Part model, mm, in its own coordinate system. Face numbers are marked on the shaded views. A direction names the side the tool comes from. Coordinates: 2 decimals unless noted, no trailing zeros. Order: outer loops, then holes, each group sorted by start corner. A loop starts at its lowest first (then second) coordinate and runs counter-clockwise, first axis right, second up.
1) Cut at B-B (x = -20.5). List the corners of the cut face in (y, z) (3 decimals), and give its area (3 significant figures).
2) Cut at D-D (x = -5.5). List the corners of the cut face in (y, z) (3 decimals).
3) Cut at C-C (y = 30.5). List the corners of the cut face in (x, z) (3 decimals), and give its area (3 significant figures).
4) Wall check: L1, parallel to Y at x = 12.5, z = 3; L2, parallel to Z at x = -19, y = 7; L3, parallel to X at y = 42.5, z = 4.5. Give the ranges that are in metal, low to high.
5) Mould opens along X. For the marked faces 1, 2 and 3 say: +X half, -X half, draft (parallel to the pull), parting line (faces both ways), or undercut.
6) Cut at A-A (y = -37.5). List the corners of the cut face in (x, z) (3 decimals), and give its area (3 significant figures).
7) Tool access for the marked faces 4, 5 and 6: list every direction of +Z, -Z, +X, -X, +Y, -Y with a clear straight run to the whole face (end or side of a thin tool).
8) Pin check, flat tips, straight feed: pin 1 Ø3 at (x, y) = (17.5, -5) entering from +Z (3 decimals); pin 2 Ø8 at (x, z) = (-1.5, 19) entering from -Y; pin 3 Ø1 at (y, z) = (-7.5, 24) entering from -X; pin 4 Ø12 at (x, y) = (-15.17, -34.82) entering from -Z. Stop position of each tip, or through.
```python
from build123d import *

# Parameters (mm, degrees)
F0_W      = 63.5
F0_H      = 101.6
F1_DEPTH  = 12.7
F5_DEPTH  = 6.35
F6_R      = 5.08
F8_D      = 10.16
F8_DEPTH  = 6.35
F8_TIP    = 3.0523719447
F10_D     = 15.24
F10_DEPTH = 12.7
F10_TIP   = 4.578557917
F12_DEPTH = 25.4
F13_R     = 5.08
F14_SIZE  = 1.905
F15_SIZE  = 1.905


with BuildPart() as f1:
    # F0 (on Top) → F1 (new body)
    with BuildSketch(Plane.XY):
        Rectangle(F0_W, F0_H)
    extrude(amount=F1_DEPTH)

    # F4 (on face) → F5 (join)
    with BuildSketch(Plane(origin=(-7.7671213914, -9.6767273995, 10.4118445509), x_dir=(0.8775350605, -0.3264402976, 0.3512391632), z_dir=(-0.4795124792, -0.5974042778, 0.6427876097))):
        Polygon((11.0284127295, 38.4279564023), (-4.4907014817, 5.8724405244), (24.646670238, -9.5275499275), (40.752428482, 24.2586095854), align=None)
    extrude(amount=-F5_DEPTH)

    # F6
    f6_edges = [f1.edges().sort_by_distance(p)[0] for p in [
        (3.43315, 16.768092, 38.405412),
        (29.517016, -3.313961, 39.199507),
    ]]
    fillet(f6_edges, radius=F6_R)

    # F8
    with Locations(Plane(origin=(-7.7671213914, -9.6767273995, 10.4118445509), x_dir=(0.8775350605, -0.3264402976, 0.3512391632), z_dir=(-0.4795124792, -0.5974042778, 0.6427876097))):
        with Locations((21.2519261986, 21.5889699757)):
            Hole(F8_D / 2, depth=F8_DEPTH)
            with Locations((0, 0, -(F8_DEPTH + F8_TIP / 2))):  # 118° drill point
                Cone(0, F8_D / 2, F8_TIP, mode=Mode.SUBTRACT)

    # F10
    with Locations(Plane.XY.offset(12.7)):
        with Locations((-15.1724275202, -34.8201803863)):
            Hole(F10_D / 2, depth=F10_DEPTH)
            with Locations((0, 0, -(F10_DEPTH + F10_TIP / 2))):  # 118° drill point
                Cone(0, F10_D / 2, F10_TIP, mode=Mode.SUBTRACT)

    # F11 (on face) → F12 (cut)
    with BuildSketch(Plane.XY.offset(12.7)):
        with BuildLine():
            ThreePointArc((-18.7010167369, 43.0184446276), (-23.7885681435, 37.6458278877), (-18.1468351234, 32.8584446276))
            Line((-18.1468351234, 32.8584446276), (20.4611556194, 32.8584446276))
            ThreePointArc((20.4611556194, 32.8584446276), (25.5411556194, 37.9384446276), (20.4611556194, 43.0184446276))
            Line((20.4611556194, 43.0184446276), (-18.7010167369, 43.0184446276))
        make_face()
    extrude(amount=-F12_DEPTH, mode=Mode.SUBTRACT)

    # F13
    f13_edges = [f1.edges().sort_by_distance(p)[0] for p in [
        (-31.75, 50.8, 6.35),
        (-31.75, -50.8, 6.35),
        (31.75, -50.8, 6.35),
        (31.75, 50.8, 6.35),
    ]]
    fillet(f13_edges, radius=F13_R)

    # F14
    f14_edges = [f1.edges().sort_by_distance(p)[0] for p in [
        (-31.75, 0, 12.7),
        (0, 50.8, 12.7),
        (-30.262102, 49.312102, 12.7),
        (30.262102, 49.312102, 12.7),
        (31.75, 0, 12.7),
        (30.262102, -49.312102, 12.7),
        (0, -50.8, 12.7),
        (-30.262102, -49.312102, 12.7),
    ]]
    chamfer(f14_edges, length=F14_SIZE)

    # F15
    f15_edges = [f1.edges().sort_by_distance(p)[0] for p in [
        (-31.75, 0, 0),
        (-30.262102, 49.312102, 0),
        (0, 50.8, 0),
        (30.262102, 49.312102, 0),
        (31.75, 0, 0),
        (30.262102, -49.312102, 0),
        (0, -50.8, 0),
        (-30.262102, -49.312102, 0),
    ]]
    chamfer(f15_edges, length=F15_SIZE)


solid = f1.part
```
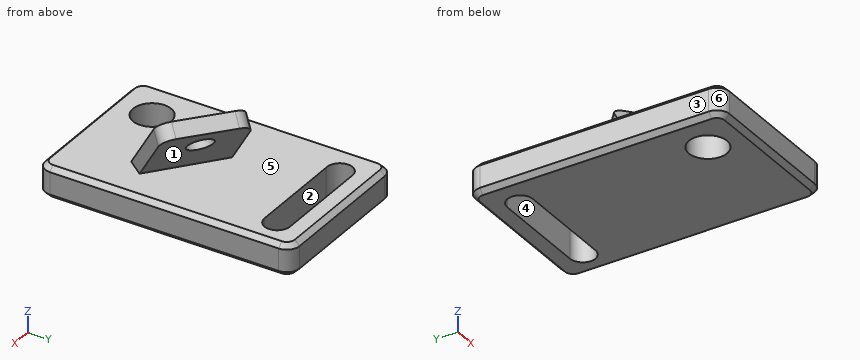
Geometry check:
1. outline: (-50.8, 1.905) - (-48.895, 0) - (-40.268, 0) - (-40.268, 12.7) - (-48.895, 12.7) - (-50.8, 10.795) - close; (-29.372, 0) - (33.156, 0) - (33.156, 12.7) - (-29.372, 12.7) - close; (42.69, 0) - (48.895, 0) - (50.8, 1.905) - (50.8, 10.795) - (48.895, 12.7) - (42.69, 12.7) - close
1. area: 1,020 mm2
2. outline: (-50.8, 1.905) - (-48.895, 0) - (32.858, 0) - (32.858, 12.7) - (1.595, 12.7) - (4.246, 15.164) - (4.652, 25.42) - (-8.957, 12.772) - (-8.846, 12.7) - (-48.895, 12.7) - (-50.8, 10.795) - close; (43.018, 0) - (48.895, 0) - (50.8, 1.905) - (50.8, 10.795) - (48.895, 12.7) - (43.018, 12.7) - close
3. outline: (-31.75, 1.905) - (-29.845, 0) - (29.845, 0) - (31.75, 1.905) - (31.75, 10.795) - (29.845, 12.7) - (-29.845, 12.7) - (-31.75, 10.795) - close
3. area: 799 mm2
4. L1: y = -50.8 to 32.86, 43.02 to 50.8
4. L2: z = 0 to 12.7
4. L3: x = -31.75 to -20.94, 22.7 to 31.75
5. face 1: +X half
5. face 2: undercut
5. face 3: -X half
6. outline: (-31.75, 1.905) - (-29.845, 0) - (-22.306, 0) - (-22.306, 12.7) - (-29.845, 12.7) - (-31.75, 10.795) - close; (-8.039, 0) - (29.845, 0) - (31.75, 1.905) - (31.75, 10.795) - (29.845, 12.7) - (-8.039, 12.7) - close
6. area: 618 mm2
7. face 4: +Z, -Z
7. face 5: none
7. face 6: +Z, -Z, -X, -Y
8. pin 1: stops at z = 35.395
8. pin 2: stops at y = -10.84
8. pin 3: stops at x = 6.82
8. pin 4: passes through
